from build123d import *

# Parameters (mm, degrees)
SKETCH1_R                = 250
SKETCH1_R_2              = 210.5
BOSS_EXTRUDE1_DEPTH      = 19.05
CUT_EXTRUDE1_DEPTH       = 355.066240272
FILLET1_R                = 1
CIRPATTERN1_COUNT        = 8
FILLET1_OF_CIRPATTERN1_R = 1


with BuildPart() as part:
    # Sketch1 → Boss-Extrude1 (new body)
    with BuildSketch(Plane(origin=(0, 0, 0), x_dir=(1, 0, 0), z_dir=(0, 1, 0))):
        with Locations(Location((0, 0, 0), (0, 0, 90))):
            Circle(SKETCH1_R)
        with Locations(Location((0, 0, 0), (0, 0, 90))):
            Circle(SKETCH1_R_2, mode=Mode.SUBTRACT)
    extrude(amount=BOSS_EXTRUDE1_DEPTH)

    # Sketch2 → Cut-Extrude1 (cut, through all)
    with BuildSketch(Plane(origin=(0, 19.05, 0), x_dir=(1, 0, 0), z_dir=(0, 1, 0))):
        with BuildLine():
            Line((6.4, 225.5), (-6.4, 225.5))
            ThreePointArc((-6.4, 225.5), (-9.6, 228.7), (-6.4, 231.9))
            Line((-6.4, 231.9), (-6.4, 250))
            Line((-6.4, 250), (6.4, 250))
            Line((6.4, 250), (6.4, 231.9))
            ThreePointArc((6.4, 231.9), (9.6, 228.7), (6.4, 225.5))
        make_face()
    cut_extrude1 = extrude(amount=-CUT_EXTRUDE1_DEPTH, mode=Mode.SUBTRACT)

    # Fillet1
    fillet1_edges = [part.edges().sort_by_distance(p)[0] for p in [
        (-6.4, 9.525, -231.9),
        (6.4, 9.525, -231.9),
    ]]
    fillet(fillet1_edges, radius=FILLET1_R)

    # CirPattern1: Cut-Extrude1 ×8 about axis
    cirpattern1_axis = Axis((0, 0, 0), (0, 1, 0))
    for i in range(1, CIRPATTERN1_COUNT):
        add(cut_extrude1.rotate(cirpattern1_axis, i * 360 / CIRPATTERN1_COUNT), mode=Mode.SUBTRACT)

    # Fillet1 of CirPattern1
    fillet1_of_cirpattern1_edges = [part.edges().sort_by_distance(p)[0] for p in [
        (-168.503545957, 9.525, -159.452579158),
        (-159.452579158, 9.525, -168.503545957),
        (-231.9, 9.525, 6.4),
        (-231.9, 9.525, -6.4),
        (-159.452579158, 9.525, 168.503545957),
        (-168.503545957, 9.525, 159.452579158),
        (6.4, 9.525, 231.9),
        (-6.4, 9.525, 231.9),
        (168.503545957, 9.525, 159.452579158),
        (159.452579158, 9.525, 168.503545957),
        (231.9, 9.525, -6.4),
        (231.9, 9.525, 6.4),
        (159.452579158, 9.525, -168.503545957),
        (168.503545957, 9.525, -159.452579158),
    ]]
    fillet(fillet1_of_cirpattern1_edges, radius=FILLET1_OF_CIRPATTERN1_R)


solid = part.part
Check sheet for the modelled part. Datum: model origin and axes. Units: mm. A direction names the side the tool comes from. Round coordinates to 2 decimals unless told otherwise and drop trailing zeros. Order: outer loops, then holes, each group sorted by start corner. A loop starts at its lowest first (then second) coordinate and runs counter-clockwise, first axis right, second up. Notation, with made-up numbers: M 11,-21.5 L 28,-21.5 A33 ccw 28,8.5 Z; hole C -19.75,-5 d3. An arc over 180 degrees is marked long. One line per item, written item: value. Start each with the question number.
1. Scan lines: line 1 along X through (y, z) = (12.25, 0); line 2 along Z through (x, y) = (58, 6.75); line 3 along X through (y, z) = (9, 128). Record each from-to range of solid material in increasing order.
2. Section check B-B on x = 0. Enter the section's corners in (y, z), and give its area (4 significant figures).
3. Gauge pin test, flat ends, axial feed: P1, Ø6, axis at y = 8, z = -140.5, coming from the -X side; P2, Ø8, axis at x = 42.5, y = 4.5, coming from the -Z side; P3, Ø4, axis at x = -3, y = 8, coming from the +Z side; P4, Ø1.5, axis at x = 184, z = -171.5, coming from the -Y side. Record the tip position at first contact, or that the pin passes through.
4. Section check A-A on z = 0. Enter the section's corners in (x, y), and give its area (4 significant figures).
5. Release check for a two-part mould opening along Z. For faces 4 (the flat face through (241, 10, 6.4)), 5 (the cylindrical face through (-231.46, 9.39, 94.48)), 6 (the cylindrical face through (-230.475, 9.392, -96.857)) record: released by +Z, released by -Z, zero draft, split by the parting line, or undercut.
6. Access from +Z, -Z, +X, -X, +Y, -Y to the whole of each face (thin tool, end or side, straight path). Record for faces 1 (the flat face through (-175.27, 9.66, 166.22)), 2 (the flat face through (-225.5, 10, 0)), 3 (the flat face through (0, 10, -225.5)).
Results found:
1. line 1: -225.5 to -210.5, 210.5 to 225.5
1. line 2: -243.18 to -202.35, 202.35 to 243.18
1. line 3: -214.75 to -167.11, 167.11 to 214.75
2. outline: M 0,-225.5 L 19.05,-225.5 L 19.05,-210.5 L 0,-210.5 Z; M 0,210.5 L 19.05,210.5 L 19.05,225.5 L 0,225.5 Z
2. area: 571.5 mm^2
3. P1: x = -208.79
3. P2: z = -247.02
3. P3: z = 225.5
3. P4: through
4. outline: M -225.5,0 L -210.5,0 L -210.5,19.05 L -225.5,19.05 Z; M 210.5,0 L 225.5,0 L 225.5,19.05 L 210.5,19.05 Z
4. area: 571.5 mm^2
5. face 4: undercut
5. face 5: released by +Z
5. face 6: released by -Z
6. face 1: +Y, -Y
6. face 2: -X, +Y, -Y
6. face 3: -Z, +Y, -Y
